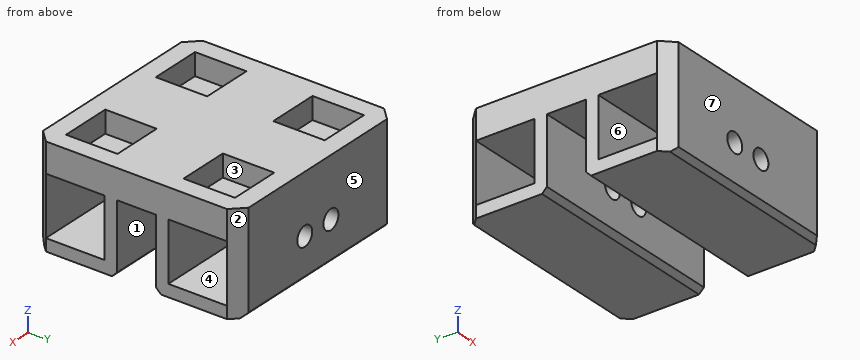
from build123d import *

# Parameters (mm, degrees)
ESQUISSE1_W               = 42
ESQUISSE1_H               = 42
BOSS_EXTRU_1_DEPTH        = 6
ESQUISSE2_W               = 42
ESQUISSE2_H               = 17
BOSS_EXTRU_3_DEPTH        = 14.5
ESQUISSE3_W               = 12
ESQUISSE3_H               = 12
ENL_V_MAT_EXTRU_3_DEPTH   = 62.141229952
ESQUISSE4_R               = 2
ENL_V_MAT_EXTRU_4_DEPTH   = 42
CHANFREIN1_SIZE           = 2.5
ESQUISSE5_W               = 10.5
ESQUISSE5_H               = 10.5
ENL_V_MAT_EXTRU_5_DEPTH   = 4.5
SYM_TRIE3_COPY_1_SKETCH_W = 10.5
SYM_TRIE3_COPY_1_SKETCH_H = 10.5
SYM_TRIE3_COPY_1_DEPTH    = 4.5
CHANFREIN2_SIZE           = 1


with BuildPart() as part:
    # Esquisse1 → Boss.-Extru.1 (new body)
    with BuildSketch(Plane.XY):
        with Locations((21, -21)):
            Rectangle(ESQUISSE1_W, ESQUISSE1_H)
    extrude(amount=BOSS_EXTRU_1_DEPTH)

    # Esquisse2 → Boss.-Extru.3 (add)
    with BuildSketch(Plane(origin=(0, 0, 0), x_dir=(-1, 0, 0), z_dir=(0, 0, -1))):
        with Locations((-21, -33.5)):
            Rectangle(ESQUISSE2_W, ESQUISSE2_H)
    boss_extru_3 = extrude(amount=BOSS_EXTRU_3_DEPTH)

    # Esquisse3 → Enlèv. mat.-Extru.3 (cut, through all)
    with BuildSketch(Plane(origin=(42, 0, 0), x_dir=(0, 0, -1), z_dir=(1, 0, 0))):
        with Locations((6, -33.5)):
            Rectangle(ESQUISSE3_W, ESQUISSE3_H)
    enl_v_mat_extru_3 = extrude(amount=-ENL_V_MAT_EXTRU_3_DEPTH, mode=Mode.SUBTRACT)

    # Symétrie1: Boss.-Extru.3, Enlèv. mat.-Extru.3 across plane
    add(boss_extru_3.mirror(Plane(origin=(0, -21, 0), x_dir=(0, 0, 1), z_dir=(0, -1, 0))))
    add(enl_v_mat_extru_3.mirror(Plane(origin=(0, -21, 0), x_dir=(0, 0, 1), z_dir=(0, -1, 0))), mode=Mode.SUBTRACT)

    # Esquisse4 → Enlèv. mat.-Extru.4 (cut)
    with BuildSketch(Plane.XZ.offset(42)):
        with Locations(Location((24.5, -6, 0), (0, 0, 270))):
            Circle(ESQUISSE4_R)
        with Locations(Location((17.5, -6, 0), (0, 0, 270))):
            Circle(ESQUISSE4_R)
    extrude(amount=-ENL_V_MAT_EXTRU_4_DEPTH, mode=Mode.SUBTRACT)

    # Chanfrein1
    chanfrein1_edges = [part.edges().sort_by_distance(p)[0] for p in [
        (42, -42, -4.25),
        (0, -42, -4.25),
        (0, 0, -4.25),
        (42, 0, -4.25),
    ]]
    chamfer(chanfrein1_edges, length=CHANFREIN1_SIZE - 0.0001)  # a hair under: the kernel refuses the full size

    # Esquisse5 → Enlèv. mat.-Extru.5 (cut)
    with BuildSketch(Plane.XY.offset(6)):
        with Locations((9, -9)):
            Rectangle(ESQUISSE5_W, ESQUISSE5_H)
    enl_v_mat_extru_5 = extrude(amount=-ENL_V_MAT_EXTRU_5_DEPTH, mode=Mode.SUBTRACT)

    # Symétrie2: Enlèv. mat.-Extru.5 across plane
    add(enl_v_mat_extru_5.mirror(Plane.ZY.offset(-21)), mode=Mode.SUBTRACT)

    # Symétrie3: Enlèv. mat.-Extru.5 across plane
    add(enl_v_mat_extru_5.mirror(Plane(origin=(0, -21, 0), x_dir=(0, 0, 1), z_dir=(0, -1, 0))), mode=Mode.SUBTRACT)

    # Symétrie3 copy 1 sketch → Symétrie3 copy 1 (cut)
    with BuildSketch(Plane(origin=(42, -42, 6), x_dir=(-1, 0, 0), z_dir=(0, 0, 1))):
        with Locations((9, -9)):
            Rectangle(SYM_TRIE3_COPY_1_SKETCH_W, SYM_TRIE3_COPY_1_SKETCH_H)
    extrude(amount=-SYM_TRIE3_COPY_1_DEPTH, mode=Mode.SUBTRACT)

    # Chanfrein2
    chanfrein2_edges = [part.edges().sort_by_distance(p)[0] for p in [
        (21, 0, -14.5),
        (21, -42, -14.5),
        (21, -25, -14.5),
        (21, -17, -14.5),
    ]]
    chamfer(chanfrein2_edges, length=CHANFREIN2_SIZE)


solid = part.part
Source: CAD feature listing. Evaluate the final solid. Frame: model axes, mm. Face numbers are marked on the shaded views. A direction names the side the tool comes from. Give positions to 0.01 mm unless a question says otherwise; leave off trailing zeros. Write each loop counter-clockwise with the first axis right and the second up, starting at its lowest first coordinate (ties: lowest second). Pieces come first, ordered by that corner, then holes. Notation, with made-up numbers: M -20.5,-14 L 7.5,-14 A18 cw 7.5,10 Z; hole C 22,-1.5 d6. An arc over 180 degrees is marked long. Answer as a JSON object with one key per item and string values.
Q1. Cut plane B-B, the plane y = -11.5. Return the cut outline in (x, z).
Geometry check:
{"outline": "M 0,-14.5 L 42,-14.5 L 42,-12 L 0,-12 Z; M 0,0 L 42,0 L 42,6 L 38.25,6 L 38.25,1.5 L 27.75,1.5 L 27.75,6 L 14.25,6 L 14.25,1.5 L 3.75,1.5 L 3.75,6 L 0,6 Z"}
Q2. Mould query, pull axis Y, two halves, no side actions, for the marked faces 5, 6 and 7. Classes: +Y half, -Y half, draft (parallel to the pull), parting line (faces both ways), or undercut.
Geometry check:
{"face 5": "+Y half", "face 6": "undercut", "face 7": "-Y half"}
Q3. Access query for the marked faces 1, 2, 3 and 4. Directions: +Z, -Z, +X, -X, +Y, -Y. A direction counts if a zero-diameter tool reaches every point of the face in a straight line with its end or side. Return the directions, or none.
Geometry check:
{"face 1": "-Z, +X, -X", "face 2": "+Z, -Z, +X, +Y", "face 3": "+Z", "face 4": "+X, -X"}
Q4. Cut plane A-A, the plane z = 2.5. Return the cut outline in (x, y).
Geometry check:
{"outline": "M 0,-39.5 L 2.5,-42 L 39.5,-42 L 42,-39.5 L 42,-2.5 L 39.5,0 L 2.5,0 L 0,-2.5 Z; hole M 3.75,-38.25 L 14.25,-38.25 L 14.25,-27.75 L 3.75,-27.75 Z; hole M 3.75,-14.25 L 14.25,-14.25 L 14.25,-3.75 L 3.75,-3.75 Z; hole M 27.75,-38.25 L 38.25,-38.25 L 38.25,-27.75 L 27.75,-27.75 Z; hole M 27.75,-14.25 L 38.25,-14.25 L 38.25,-3.75 L 27.75,-3.75 Z"}
Q5. Cut plane C-C, the plane x = 8.5. Return the cut outline in (y, z).
Geometry check:
{"outline": "M -42,-13.5 L -41,-14.5 L -26,-14.5 L -25,-13.5 L -25,0 L -17,0 L -17,-13.5 L -16,-14.5 L -1,-14.5 L 0,-13.5 L 0,6 L -3.75,6 L -3.75,1.5 L -14.25,1.5 L -14.25,6 L -27.75,6 L -27.75,1.5 L -38.25,1.5 L -38.25,6 L -42,6 Z; hole M -39.5,-12 L -27.5,-12 L -27.5,0 L -39.5,0 Z; hole M -14.5,-12 L -2.5,-12 L -2.5,0 L -14.5,0 Z"}
Q6. Ray query, line 1 along Y through (x, z) = (31.5, 5); line 2 along X through (y, z) = (-25.5, -6); line 3 along Y through (x, z) = (31, -0.25). Return the intervals inside material, ascending.
Geometry check:
{"line 1": "y = -42 to -38.25, -27.75 to -14.25, -3.75 to 0", "line 2": "x = 0 to 15.5, 19.5 to 22.5, 26.5 to 42", "line 3": "y = -42 to -39.5, -27.5 to -25, -17 to -14.5, -2.5 to 0"}
Q7. Cut plane D-D, the plane z = -2.5. Count the separate pieces of the cut face and the enclosed holes in it, then the cut area to 4 significant figures.
Geometry check:
{"separate pieces": "4", "enclosed holes": "0", "area": "407.5 mm^2"}
